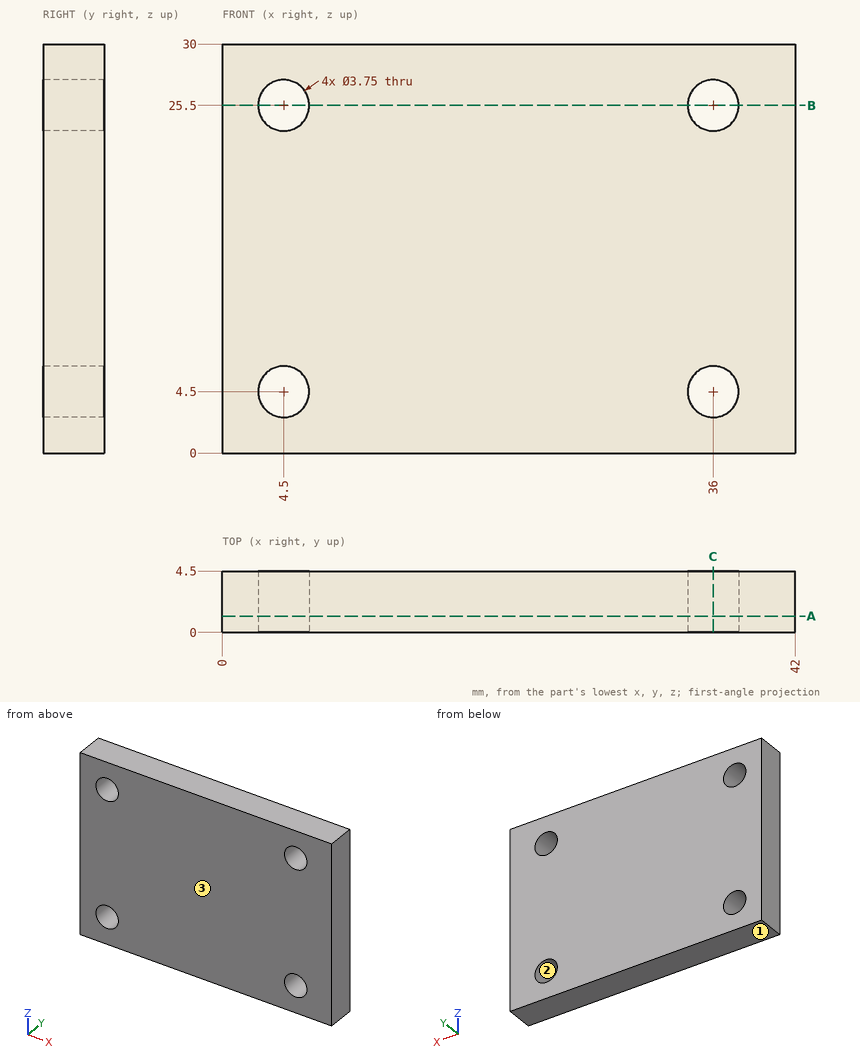
Check sheet for the drawn part. Datum: minimum x, y, z corner. Units: mm. Give positions to 0.01 mm unless a question says otherwise; leave off trailing zeros. Order: outer loops, then holes, each group sorted by start corner. A loop starts at its lowest first (then second) coordinate and runs counter-clockwise, first axis right, second up. Notation, with made-up numbers: (-35, -11.75) -> (-18, -11.75) arc R30 ccw to (-18, 13.25) -> close; hole circle Ø11 at (-34.75, -39.5). An arc over 180 degrees is marked (long way). Answer as CSV lines item,"result".
Q1. Sectioned sample at C-C on x = 36. Record the cut outline in (y, z) (3 decimals), plus the area to 3 significant figures.
Solutions:
outline,"(0, 0) -> (4.5, 0) -> (4.5, 2.625) -> (0, 2.625) -> close; (0, 6.375) -> (4.5, 6.375) -> (4.5, 23.625) -> (0, 23.625) -> close; (0, 27.375) -> (4.5, 27.375) -> (4.5, 30) -> (0, 30) -> close"
area,"101 mm²"
Q2. Sectioned sample at A-A on y = 1.2. Record the cut outline in (x, z) (3 decimals), plus the area to 3 significant figures.
Solutions:
outline,"(0, 0) -> (42, 0) -> (42, 30) -> (0, 30) -> close; hole circle Ø3.75 at (4.5, 4.5); hole circle Ø3.75 at (4.5, 25.5); hole circle Ø3.75 at (36, 4.5); hole circle Ø3.75 at (36, 25.5)"
area,"1,220 mm²"
Q3. Sectioned sample at B-B on z = 25.5. Record the cut outline in (x, y) (3 decimals).
Solutions:
outline,"(0, 0) -> (2.625, 0) -> (2.625, 4.5) -> (0, 4.5) -> close; (6.375, 0) -> (34.125, 0) -> (34.125, 4.5) -> (6.375, 4.5) -> close; (37.875, 0) -> (42, 0) -> (42, 4.5) -> (37.875, 4.5) -> close"
Q4. Scan lines: probe 1 along Z at (x, y) = (4.5, 1.4) (3 decimals); probe 2 along X at (y, z) = (2.4, 25.5) (3 decimals); probe 3 along X at (y, z) = (2.85, 25). Record each from-to range of solid material in increasing order.
Solutions:
probe 1,"z = 0 to 2.625, 6.375 to 23.625, 27.375 to 30"
probe 2,"x = 0 to 2.625, 6.375 to 34.125, 37.875 to 42"
probe 3,"x = 0 to 2.69, 6.31 to 34.19, 37.81 to 42"
Q5. Release check for a two-part mould opening along Z. For the marked faces 1, 2 and 3 record: +Z half, -Z half, draft (parallel to the pull), parting line (faces both ways), or undercut.
Solutions:
face 1,"-Z half"
face 2,"undercut"
face 3,"draft"
